Geometry check sheet. Reference: the model listing, model coordinates, mm. A direction names the side the tool comes from. Round coordinates to 2 decimals unless told otherwise and drop trailing zeros. Loops run counter-clockwise (first coordinate to the right, second up) from the corner with the lowest first, then second, coordinate; pieces in that order, holes last. Notation, with made-up numbers: M 52.5,75.25 L 72.5,75.25 A25 ccw 72.5,103.25 Z; hole C 58,67 d9. An arc over 180 degrees is marked long. Write item = value, one per line.
from build123d import *

# Parameters (mm, degrees)
F0_R     = 1.905
F1_DEPTH = 12.7


with BuildPart() as f1:
    # F0 (on Top) → F1 (new body)
    with BuildSketch(Plane.XY):
        with BuildLine():
            Line((3.466116, 1.165293), (2.111037, 2.371528))
            ThreePointArc((2.111037, 2.371528), (-2.967341, 1.129385), (0, -3.175))
            Line((0, -3.175), (4.7752, -3.175))
            ThreePointArc((4.7752, -3.175), (7.801505, -0.960261), (6.605779, 2.594148))
            ThreePointArc((6.605779, 2.594148), (6.270566, 2.61704), (6.096, 2.329955))
            Line((6.096, 2.329955), (6.096, 1.151996))
            ThreePointArc((6.096, 1.151996), (4.766339, -1.752578), (3.466116, 1.165293))
        make_face()
        Circle(F0_R, mode=Mode.SUBTRACT)
    extrude(amount=F1_DEPTH)


solid = f1.part
(1) Sectioned sample at A-A on z = 3.75. Record the cut outline in (x, y) (3 decimals).
Result set:
outline = M 0,-3.175 L 4.775,-3.175 A3.175 ccw 6.606,2.594 A0.323 ccw 6.096,2.33 L 6.096,1.152 A1.753 cw long 3.466,1.165 L 2.111,2.372 A3.175 ccw long Z; hole C 0,0 d3.81
(2) Tool access check on faces 4 (the flat face through (6.096, 2, 6)), 5 (the flat face through (2, -1, 12.7)). Record the directions out of +Z, -Z, +X, -X, +Y, -Y that give a thin tool (end or side, any length) a straight path to the whole face; none if there is none.
Result set:
face_4 = +Z, -Z, +Y
face_5 = +Z, +X, -X, +Y, -Y
(3) Material ranges on line 1 along X through (y, z) = (1, 11.75); line 2 along X through (y, z) = (-1.5, 12.25); line 3 along Y through (x, z) = (4.75, 8.5) (3 decimals), recorded low to high. Write a range as from..to.
Result set:
line_1 = -3.01..-1.62, 1.62..3.34, 6.21..7.79
line_2 = -2.8..-1.17, 1.17..3.87, 5.68..7.57
line_3 = -3.175..-1.752
(4) Sectioned sample at C-C on x = -1. Record the cut outline in (y, z).
Result set:
outline = M -3.01,0 L -1.62,0 L -1.62,12.7 L -3.01,12.7 Z; M 1.62,0 L 3.01,0 L 3.01,12.7 L 1.62,12.7 Z
(5) Sectioned sample at B-B on y = 0. Record the cut outline in (x, z) (3 decimals), then the cut area to 3 significant figures.
Result set:
outline = M -3.175,0 L -1.905,0 L -1.905,12.7 L -3.175,12.7 Z; M 1.905,0 L 3.023,0 L 3.023,12.7 L 1.905,12.7 Z; M 6.528,0 L 7.95,0 L 7.95,12.7 L 6.528,12.7 Z
area = 48.4 mm2
(6) Release check for a two-part mould opening along Y. For faces 1 (the flat face through (2, -3.175, 6)), 2 (the cylindrical face through (-0.41, -1.86, 6.26)), 3 (the cylindrical face through (7.784, -1.014, 6.261)) record: released by +Y, released by -Y, zero draft, split by the parting line, or undercut.
Result set:
face_1 = released by -Y
face_2 = undercut
face_3 = split by the parting line
(7) Depth check by flat-ended pin: pin 1 Ø3 at (x, z) = (5.5, 8.5) entering from +Y; pin 2 Ø2 at (x, y) = (0.5, 1.5) entering from -Z; pin 3 Ø1.3 at (y, z) = (1.5, 9) entering from -X; pin 4 Ø2.5 at (x, y) = (0, 0) entering from +Z. Enter the tip coordinate at first touch or a pass-through.
Result set:
pin_1 = 2.65
pin_2 = 0
pin_3 = -3.06
pin_4 = through
(8) Sectioned sample at D-D on y = -1.5. Record the cut outline in (x, z).
Result set:
outline = M -2.8,0 L -1.17,0 L -1.17,12.7 L -2.8,12.7 Z; M 1.17,0 L 3.87,0 L 3.87,12.7 L 1.17,12.7 Z; M 5.68,0 L 7.57,0 L 7.57,12.7 L 5.68,12.7 Z
